from build123d import *

# Parameters (mm, degrees)
F0_R          = 17.7524356155
F0_W          = 7.8417137265
F0_H          = 11.7625724524
F1_DEPTH      = 12.7
F0_W_2        = 6.861500442
F2_DEPTH      = 12.7
F3_DEPTH      = 12.7
F4_DEPTH      = 12.7
F5_DEPTH      = 12.7
F5_DEPTH_BACK = 12.7


with BuildPart() as f1:
    # F0 (on Front) → F1 (new body)
    with BuildSketch(Plane.XZ):
        with BuildLine():
            ThreePointArc((52.2818670696, 21.9389039537), (52.3286615447, 22.7927192156), (52.3442666326, 23.6476734281))
            ThreePointArc((52.3442666326, 23.6476734281), (28.1944509327, 47.0644925256), (5.5328658292, 22.2046136927))
            Line((5.5328658292, 22.2046136927), (12.3917076344, 7.0402779271))
            ThreePointArc((12.3917076344, 7.0402779271), (29.1464973283, 0.2208610805), (45.764060769, 7.3681689029))
            Line((45.764060769, 7.3681689029), (52.2818670696, 21.9389039537))
        make_face()
        with Locations((28.9163235575, 23.6476734281)):
            Circle(F0_R, mode=Mode.SUBTRACT)
        with BuildLine():
            ThreePointArc((45.764060769, 7.3681689029), (29.1464973283, 0.2208610805), (12.3917076344, 7.0402779271))
            Line((12.3917076344, 7.0402779271), (18.6240747571, -6.7389737815))
            Line((18.6240747571, -6.7389737815), (39.4536294043, -6.7389737815))
            Line((39.4536294043, -6.7389737815), (45.764060769, 7.3681689029))
        make_face()
        Polygon((39.4536294043, -6.7389737815), (18.6240747571, -6.7389737815), (18.6240747571, -15.0707960129), (25.4855751991, -15.0707960129), (33.3272889256, -15.0707960129), (39.4536294043, -15.0707960129), align=None)
        with Locations((29.4064320624, -20.9520822391)):
            Rectangle(F0_W, F0_H)
    extrude(amount=F1_DEPTH)

    # F0 (on Front) → F2 (join)
    with BuildSketch(Plane.XZ):
        with BuildLine():
            ThreePointArc((52.2818670696, 21.9389039537), (52.3286615447, 22.7927192156), (52.3442666326, 23.6476734281))
            ThreePointArc((52.3442666326, 23.6476734281), (28.1944509327, 47.0644925256), (5.5328658292, 22.2046136927))
            Line((5.5328658292, 22.2046136927), (12.3917076344, 7.0402779271))
            ThreePointArc((12.3917076344, 7.0402779271), (29.1464973283, 0.2208610805), (45.764060769, 7.3681689029))
            Line((45.764060769, 7.3681689029), (52.2818670696, 21.9389039537))
        make_face()
        with Locations((28.9163235575, 23.6476734281)):
            Circle(F0_R, mode=Mode.SUBTRACT)
        with BuildLine():
            Line((12.3917076344, 7.0402779271), (5.5328658292, 22.2046136927))
            ThreePointArc((5.5328658292, 22.2046136927), (7.5702968676, 13.992847625), (12.3917076344, 7.0402779271))
        make_face()
        with BuildLine():
            ThreePointArc((45.764060769, 7.3681689029), (50.3021498595, 14.0813287702), (52.2818670696, 21.9389039537))
            Line((52.2818670696, 21.9389039537), (45.764060769, 7.3681689029))
        make_face()
        with BuildLine():
            ThreePointArc((45.764060769, 7.3681689029), (29.1464973283, 0.2208610805), (12.3917076344, 7.0402779271))
            Line((12.3917076344, 7.0402779271), (18.6240747571, -6.7389737815))
            Line((18.6240747571, -6.7389737815), (39.4536294043, -6.7389737815))
            Line((39.4536294043, -6.7389737815), (45.764060769, 7.3681689029))
        make_face()
        Polygon((39.4536294043, -6.7389737815), (18.6240747571, -6.7389737815), (18.6240747571, -15.0707960129), (25.4855751991, -15.0707960129), (33.3272889256, -15.0707960129), (39.4536294043, -15.0707960129), align=None)
        Polygon((39.6986864507, -6.7389737815), (39.4536294043, -6.7389737815), (39.4536294043, -15.0707960129), (33.3272889256, -15.0707960129), (33.3272889256, -26.8333684653), (39.6986864507, -26.8333684653), align=None)
        with Locations((22.0548249781, -20.9520822391)):
            Rectangle(F0_W_2, F0_H)
        with Locations((29.4064320624, -20.9520822391)):
            Rectangle(F0_W, F0_H)
    extrude(amount=-F2_DEPTH)

    # F3 (add): a face of the model
    f3_faces = [f1.faces().sort_by_distance(p)[0] for p in [
        (28.6947474354, 12.7, 46.1994273244),
    ]]
    extrude(f3_faces, amount=F3_DEPTH)

    # F4 (add): faces of the model
    f4_faces = [f1.faces().sort_by_distance(p)[0] for p in [
        (36.5942272767, 0, -20.6856164164),
        (22.0548249781, 0, -20.9520822391),
    ]]
    extrude(f4_faces, amount=-F4_DEPTH)

    # F5 (cut, two sides): faces of the model
    f5_faces = [f1.faces().sort_by_distance(p)[0] for p in [
        (36.5942272767, 0, -20.6856164164),
        (22.0548249781, 0, -20.9520822391),
    ]]
    extrude(f5_faces, amount=F5_DEPTH, mode=Mode.SUBTRACT)
    extrude(f5_faces, amount=-F5_DEPTH_BACK, mode=Mode.SUBTRACT)


solid = f1.part
Verification items for the finished model (mm, model axes). A direction names the side the tool comes from. Give positions to 0.01 mm unless a question says otherwise; leave off trailing zeros. Write each loop counter-clockwise with the first axis right and the second up, starting at its lowest first coordinate (ties: lowest second). Pieces come first, ordered by that corner, then holes. Notation, with made-up numbers: M 48.5,74.25 L 88.5,74.25 A18 cw 88.5,85.25 Z; hole C 79.5,65.25 d10. An arc over 180 degrees is marked long. Put each result on its own line as item: value. Start each with the question number.
1. Draft check along X on faces 4 (the face through (33.327, 0, -21)), 5 (the face through (8, 0, 14)), 6 (the face through (15.832, 6.617, 35.646)). Enter one of: +X half, -X half, draft (parallel to the pull), parting line (faces both ways), or undercut.
2. Go/stop test with flat-tipped pins: pin 1 Ø5 at (x, y) = (36.5, -2.5) entering from -Z; pin 2 Ø10 at (y, z) = (17.5, -19) entering from +X; pin 3 Ø8 at (y, z) = (-9, 3.5) entering from -X. Record where each tip stops, or that it passes through.
3. Scan lines: line 1 along X through (y, z) = (19, -10); line 2 along Z through (x, y) = (42, 9.5); line 3 along X through (y, z) = (5.5, 20). Record each from-to range of solid material in increasing order. Write a range as [from, to].
4. Section check A-A (z = 37). Record the cut outline in (x, y), and give its area (3 significant figures).
5. Section check C-C (y = 18). Record the cut outline in (x, z).
6. Set-up check for faces 1 (the face through (22, 12.7, -21)), 2 (the face through (49, 0, 14)), 3 (the face through (39.699, 19, -17)): record each of +Z, -Z, +X, -X, +Y, -Y from which the full face is reachable in a straight line by a thin tool's end or side.
7. Section check D-D (x = 22.5). Record the cut outline in (y, z), and give its area (3 significant figures).
8. Section check B-B (x = 31.5). Record the cut outline in (y, z).
Answer list:
1. face 4: +X half
1. face 5: draft
1. face 6: undercut
2. pin 1: z = -15.07
2. pin 2: x = 39.7
2. pin 3: x = 12.18
3. line 1: [18.62, 39.7]
3. line 2: [-1.05, 11.65], [35.65, 43.08]
3. line 3: [5.77, 11.54], [46.29, 52.06]
4. outline: M 9.67,-12.7 L 17.22,-12.7 L 17.22,25.4 L 9.67,25.4 Z; M 40.62,-12.7 L 48.17,-12.7 L 48.17,25.4 L 40.62,25.4 Z
4. area: 575 mm2
5. outline: M 12.39,7.04 L 18.62,-6.74 L 18.62,-26.83 L 39.7,-26.83 L 39.7,-6.74 L 39.45,-6.74 L 45.76,7.37 A23.43 ccw long Z; hole C 28.92,23.65 d35.5
6. face 1: -Z, -X, -Y
6. face 2: -Z, +X, -Y
6. face 3: -Z, +X, +Y, -Y
7. outline: M -12.7,-15.07 L 12.7,-15.07 L 12.7,-26.83 L 25.4,-26.83 L 25.4,7.1 L -12.7,7.1 Z; M -12.7,40.2 L 25.4,40.2 L 25.4,46.18 L -12.7,46.18 Z
7. area: 1,220 mm2
8. outline: M -12.7,-26.83 L 25.4,-26.83 L 25.4,6.08 L -12.7,6.08 Z; M -12.7,41.21 L 25.4,41.21 L 25.4,46.93 L -12.7,46.93 Z
